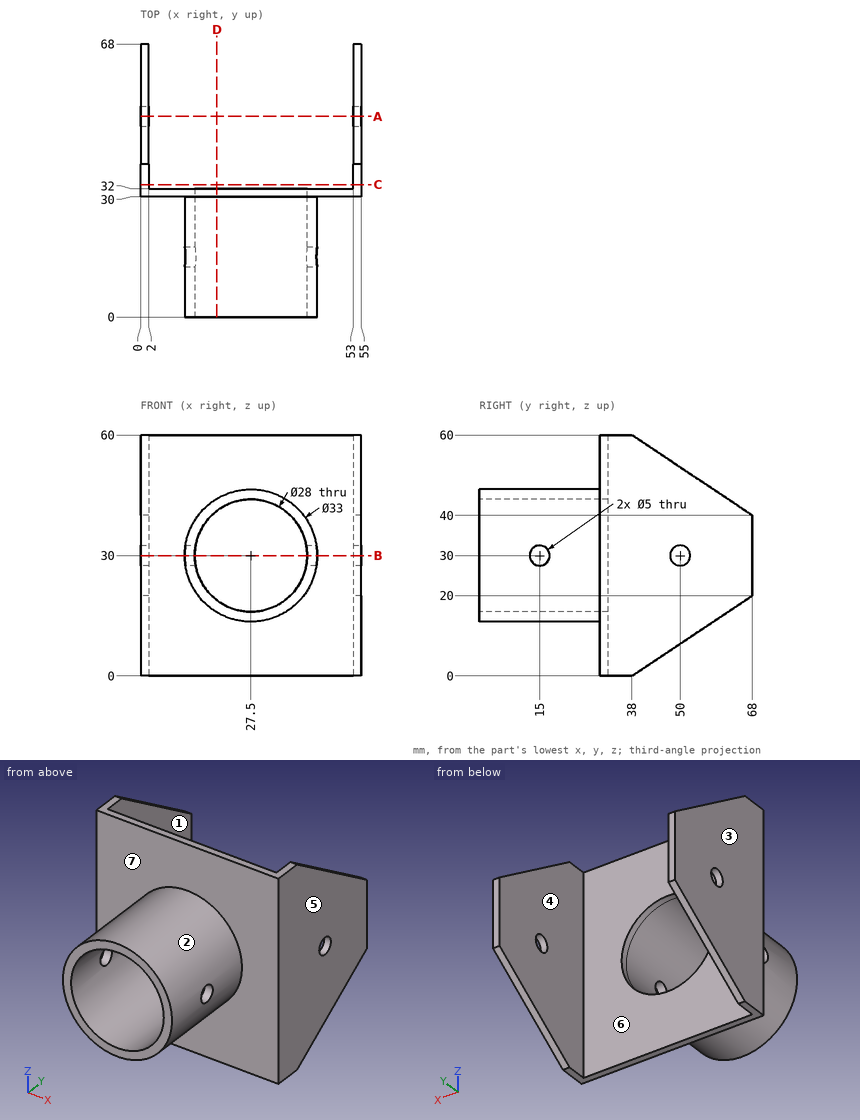
Drawing for the job (mm, zero at the part's lowest x, y, z). A direction names the side the tool comes from. Round coordinates to 2 decimals unless told otherwise and drop trailing zeros. Write each loop counter-clockwise with the first axis right and the second up, starting at its lowest first coordinate (ties: lowest second). Pieces come first, ordered by that corner, then holes. Notation, with made-up numbers: (59.25, 14) - (107.25, 14) arc R22 cw to (107.25, 23) - close; hole circle Ø9 at (38.25, 50). An arc over 180 degrees is marked (long way). Use CSV: the item, a comma, the result in double quotes.
(1) Band-saw the part on D-D (x = 19). Write the cut outline in (y, z).
Response:
outline,"(0, 15.86) - (30, 15.86) - (30, 0) - (32, 0) - (32, 18.88) - (0, 18.88) - close; (0, 41.12) - (32, 41.12) - (32, 60) - (30, 60) - (30, 44.14) - (0, 44.14) - close"
(2) Band-saw the part on B-B (z = 30). Give the number of separate pieces and of enclosed holes in the cut face, plus the area to 3 significant figures.
Response:
separate pieces,"6"
enclosed holes,"0"
area,"303 mm²"
(3) Band-saw the part on C-C (y = 33). Write the cut outline in (x, z).
Response:
outline,"(0, 0) - (2, 0) - (2, 60) - (0, 60) - close; (53, 0) - (55, 0) - (55, 60) - (53, 60) - close"
(4) Mould opens along X. For the marked faces 1, 2, 3 and 4 say: pulls with the +X half, pulls with the -X half, needs draft (parallel to the pull), parting line crosses it, or undercut.
Response:
face 1,"undercut"
face 2,"parting line crosses it"
face 3,"pulls with the -X half"
face 4,"undercut"
(5) Band-saw the part on A-A (y = 50). Write the cut outline in (x, z).
Response:
outline,"(0, 8) - (2, 8) - (2, 27.5) - (0, 27.5) - close; (0, 32.5) - (2, 32.5) - (2, 52) - (0, 52) - close; (53, 8) - (55, 8) - (55, 27.5) - (53, 27.5) - close; (53, 32.5) - (55, 32.5) - (55, 52) - (53, 52) - close"
(6) Pin check, flat tips, straight feed: P1, Ø4, axis at y = 15, z = 30, coming from the -X side; P2, Ø4, axis at y = 19, z = 36.5, coming from the -X side; P3, Ø12, axis at y = 9.5, z = 14.5, coming from the -X side; P4, Ø12, axis at y = 17, z = 10.5, coming from the -X side. Stop position of each tip, or through.
Response:
P1,"through"
P2,"x = 11.63"
P3,"x = 14.01"
P4,"x = 18.01"
(7) 3-axis set-ups, long thin cutter, end or side, ignore diameter. For the marked faces 5, 6 and 7: which of +Z, -Z, +X, -X, +Y, -Y reach the whole face in a straight line?
Response:
face 5,"+Z, -Z, +X, +Y, -Y"
face 6,"+Z, -Z, +Y"
face 7,"-Y"
(8) Wall check: line 1 (Y direction, x = 54.55, z = 30); line 2 (X direction, y = 57, z = 33); line 3 (Z direction, x = 27, y = 12). Give the ranges that are in metal, low to high.
Response:
line 1,"30 to 47.5, 52.5 to 68"
line 2,"0 to 2, 53 to 55"
line 3,"13.51 to 16.01, 43.99 to 46.49"
